from build123d import *

# Parameters (mm, degrees)
F0_R     = 5.7785
F1_DEPTH = 15.875
F2_DEPTH = 5.08
F3_D     = 5.08
F5_R     = 5.7785
F5_W     = 7.112
F5_H     = 7.112
F6_DEPTH = 8.382


with BuildPart() as f1:
    # F0 (on Top) → F1 (new body)
    with BuildSketch(Plane.XY):
        Circle(F0_R)
        Polygon((2.851977, 4.267348), (5.12162, -0.336211), (2.269643, -4.603559), (-2.851977, -4.267348), (-5.12162, 0.336211), (-2.269643, 4.603559), align=None, mode=Mode.SUBTRACT)
        Polygon((2.269643, -4.603559), (5.12162, -0.336211), (2.851977, 4.267348), (-2.269643, 4.603559), (-5.12162, 0.336211), (-2.851977, -4.267348), align=None)
    extrude(amount=F1_DEPTH)

    # F0 (on Top) → F2 (cut)
    with BuildSketch(Plane.XY):
        Polygon((2.269643, -4.603559), (5.12162, -0.336211), (2.851977, 4.267348), (-2.269643, 4.603559), (-5.12162, 0.336211), (-2.851977, -4.267348), align=None)
    extrude(amount=F2_DEPTH, mode=Mode.SUBTRACT)

    # F3 (through all)
    with Locations(Plane(origin=(0, 0, 0), x_dir=(1, 0, 0), z_dir=(0, 0, -1))):
        with Locations((0, 0)):
            Hole(F3_D / 2)

    # F5 (on face) → F6 (join)
    with BuildSketch(Plane.XY.offset(15.875)):
        Circle(F5_R)
        Rectangle(F5_W, F5_H, mode=Mode.SUBTRACT)
    extrude(amount=F6_DEPTH)


solid = f1.part
Read the model definition and answer for the solid it produces. Units are mm, in the model's axes. A direction names the side the tool comes from. Round coordinates to 2 decimals unless told otherwise and drop trailing zeros. Order: outer loops, then holes, each group sorted by start corner. A loop starts at its lowest first (then second) coordinate and runs counter-clockwise, first axis right, second up. Notation, with made-up numbers: (-20.5, 15.25) - (-13.5, 15.25) arc R18 ccw to (-13.5, 33.25) - close; hole circle Ø10 at (64.25, -27). An arc over 180 degrees is marked (long way). Use one line per item in the form item = value. Start each with the question number.
(1) The part is cut by section A-A (z = 4.75). Give the vertices of the cut face in (x, y).
(2) The part is cut by section D-D (z = 19.75). Give the vertices of the cut face in (x, y).
(3) The part is cut by section B-B (y = -1.5). Give the vertices of the cut face in (x, z) (3 decimals), then the cut area to 3 significant figures.
(4) For faces 4 (the face through (0, -3.556, 20)), 5 (the face through (0.33, -2.52, 10.55)), 6 (the face through (-3.676, 2.5, 2.504)), determine the directions among +Z, -Z, +X, -X, +Y, -Y from which every point of the face is accessible in a straight line to the end or side of a thin tool.
(5) The part is cut by section C-C (x = 0). Give the vertices of the cut face in (y, z) (1 decimal), then the cut area to 3 significant figures.
(6) Determine the mould class of faces 1 (the face through (0, -4, 24.257)), 2 (the face through (-4.003, -1.933, 2.504)), 3 (the face through (3.11, 4.87, 11.96)) for opening direction X: +X half, -X half, draft (parallel to the pull), parting line (faces both ways), or undercut.
(7) Find the intervals of material crossed by line 1 along Y through (x, z) = (0.25, 20); line 2 along Y through (x, z) = (1.5, 5.25); line 3 along Z through (x, y) = (4, -0.25), in increasing order. Write a range as from..to.
(8) Flat-ended cylindrical pins translate along their axes: pin 1 Ø5 at (y, z) = (-4.5, 6.5) entering from +X; pin 2 Ø1.5 at (x, z) = (2, 3.5) entering from +Y; pin 3 Ø2 at (y, z) = (2, 19) entering from -X. Find the tip coordinate at first contact, or state that the pin passes through.
Checked values:
q1.outline = circle Ø11.56 at (0, 0); hole (-5.12, 0.34) - (-2.85, -4.27) - (2.27, -4.6) - (5.12, -0.34) - (2.85, 4.27) - (-2.27, 4.6) - close
q2.outline = circle Ø11.56 at (0, 0); hole (-3.56, -3.56) - (3.56, -3.56) - (3.56, 3.56) - (-3.56, 3.56) - close
q3.outline = (-5.58, 0) - (-4.216, 0) - (-4.216, 5.08) - (-2.05, 5.08) - (-2.05, 15.875) - (-3.556, 15.875) - (-3.556, 24.257) - (-5.58, 24.257) - close; (2.05, 5.08) - (4.344, 5.08) - (4.344, 0) - (5.58, 0) - (5.58, 24.257) - (3.556, 24.257) - (3.556, 15.875) - (2.05, 15.875) - close
q3.area = 123 mm^2
q4.face_4 = +Z
q4.face_5 = +Z, -Z
q4.face_6 = -Z
q5.outline = (-5.8, 0) - (-4.5, 0) - (-4.5, 5.1) - (-2.5, 5.1) - (-2.5, 15.9) - (-3.6, 15.9) - (-3.6, 24.3) - (-5.8, 24.3) - close; (2.5, 5.1) - (4.5, 5.1) - (4.5, 0) - (5.8, 0) - (5.8, 24.3) - (3.6, 24.3) - (3.6, 15.9) - (2.5, 15.9) - close
q5.area = 121 mm^2
q6.face_1 = draft
q6.face_2 = undercut
q6.face_3 = parting line
q7.line_1 = -5.77..-3.56, 3.56..5.77
q7.line_2 = -5.58..-2.05, 2.05..5.58
q7.line_3 = 5.08..24.26
q8.pin_1 = 5.42
q8.pin_2 = 5.64
q8.pin_3 = -5.69
